```python
from build123d import *

# Parameters (mm, degrees)
SKETCH029_W     = 12.6
SKETCH029_H     = 5.7
PAD009_DEPTH    = 6.5
SKETCH030_R     = 1
POCKET025_DEPTH = 5.701
PAD010_DEPTH    = 5.7


with BuildPart() as part:
    # Sketch029 → Pad009 (new body)
    with BuildSketch(Plane.XY):
        with Locations((6.3, 2.85)):
            Rectangle(SKETCH029_W, SKETCH029_H)
    extrude(amount=PAD009_DEPTH)

    # Sketch030 (on Face1 of Pad009) → Pocket025 (cut, through all)
    with BuildSketch(Plane(origin=(0, 5.7, 0), x_dir=(-1, 0, 0), z_dir=(0, 1, 0))):
        with Locations((-9.55, 1.5)):
            Circle(SKETCH030_R)
        with Locations((-3.05, 1.5)):
            Circle(SKETCH030_R)
    extrude(amount=-POCKET025_DEPTH, mode=Mode.SUBTRACT)

    # Sketch031 (on Face1 of Pocket025) → Pad010 (join)
    with BuildSketch(Plane(origin=(0, 5.7, 0), x_dir=(-1, 0, 0), z_dir=(0, 1, 0))):
        Polygon((-11.6, 6.5), (1.6, 8), (1.611291, 7.900639), (-10.714336, 6.5), align=None)
    extrude(amount=-PAD010_DEPTH)


solid = part.part
```
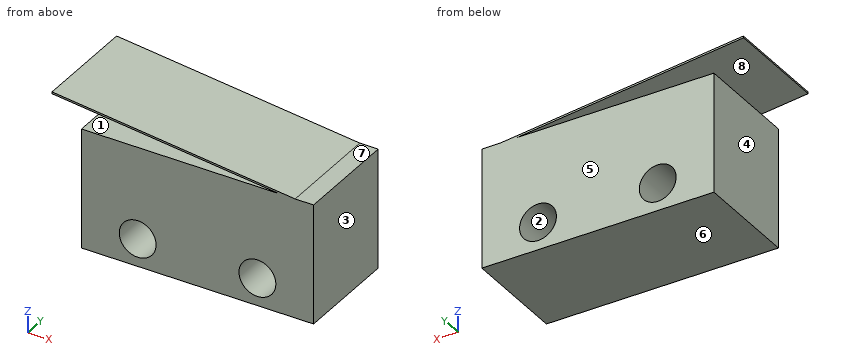
Here's how the part is built. I have some questions about the finished solid (model axes, mm). Face numbers are marked on the shaded views. A direction names the side the tool comes from. Coordinates: 2 decimals unless noted, no trailing zeros. Order: outer loops, then holes, each group sorted by start corner. A loop starts at its lowest first (then second) coordinate and runs counter-clockwise, first axis right, second up. Notation, with made-up numbers: (49, -31) - (82, -31) arc R17 cw to (82, 1) - close; hole circle Ø6 at (-36, -34). An arc over 180 degrees is marked (long way). One line per question, with ' | ' between items.
(1) If we mould it in two halves opening along X, with no side actions, what happens to the marked faces 1, 2 and 3? For each: pulls with the +X half, pulls with the -X half, needs draft (parallel to the pull), parting line crosses it, or undercut.
Report:
face 1: needs draft | face 2: undercut | face 3: pulls with the +X half
(2) If I drill on L1, parallel to X at y = 2.65, z = 1; L2, parallel to X at y = 3.85, z = 4; L3, parallel to X at y = 5.4, z = 2.25, over which ranges is the centre line in solid material (lowest first)?
Report:
L1: x = 0 to 2.18, 3.92 to 8.68, 10.42 to 12.6 | L2: x = 0 to 12.6 | L3: x = 0 to 2.39, 3.71 to 8.89, 10.21 to 12.6
(3) For the marked faces 4, 5, 6, 7 and 8, which set-ups out of +Z, -Z, +X, -X, +Y, -Y let a thin tool reach every point of the face, with its end or its side?
Report:
face 4: -Z, -X, +Y, -Y | face 5: +Z, -Z, +X, -X, +Y | face 6: -Z, +X, -X, +Y, -Y | face 7: +Z, +X, +Y, -Y | face 8: -X, +Y, -Y
(4) Suppose I cut it at C-C on x = 9.55. List the corners of the cut face in (y, z) for me.
Report:
outline: (0, 0) - (5.7, 0) - (5.7, 0.5) - (0, 0.5) - close; (0, 2.5) - (5.7, 2.5) - (5.7, 6.5) - (0, 6.5) - close; (0, 6.63) - (5.7, 6.63) - (5.7, 6.73) - (0, 6.73) - close
(5) Suppose I cut it at D-D on z = 5. List the corners of the cut face in (x, y) for me, and give its area (3 significant figures).
Report:
outline: (0, 0) - (12.6, 0) - (12.6, 5.7) - (0, 5.7) - close | area: 71.8 mm2
(6) Suppose I cut it at B-B on x = 0.5. List the corners of the cut face in (y, z) for me.
Report:
outline: (0, 0) - (5.7, 0) - (5.7, 6.5) - (0, 6.5) - close; (0, 7.66) - (5.7, 7.66) - (5.7, 7.76) - (0, 7.76) - close
(7) Will these pins go through, and if not, where does the flat tip stop? pin 1 (1.5 mm diameter, centred on x = 10, y = 2, fed in from +Z); pin 2 (1.1 mm diameter, centred on x = 12.5, y = 3, fed in from +Z); pin 3 (2.5 mm diameter, centred on x = 3.05, z = 1.5, fed in from -Y); pin 4 (3 mm diameter, centred on y = 3, z = 3, fed in from -X).
Report:
pin 1: stops at z = 6.77 | pin 2: stops at z = 6.5 | pin 3: stops at y = 0 | pin 4: stops at x = 0
(8) Suppose I cut it at A-A on y = 0.5. List the corners of the cut face in (x, z) for me, and give its area (3 significant figures).
Report:
outline: (-1.61, 7.9) - (10.71, 6.5) - (0, 6.5) - (0, 0) - (12.6, 0) - (12.6, 6.5) - (11.6, 6.5) - (-1.6, 8) - close; hole circle Ø2 at (3.05, 1.5); hole circle Ø2 at (9.55, 1.5) | area: 76.9 mm2
